from build123d import *

# Parameters (mm, degrees)
SALIENTE_EXTRUIR1_DEPTH = 5
CROQUIS3_W              = 50
CROQUIS3_H              = 80
CORTAR_EXTRUIR2_DEPTH   = 10
CHAFL_N1_SIZE           = 5
REDONDEO1_R             = 3
CROQUIS4_R              = 2.25
CORTAR_EXTRUIR3_DEPTH   = 5
CROQUIS5_R              = 30
CORTAR_EXTRUIR4_DEPTH   = 327.750669471


with BuildPart() as part:
    # Croquis1 → Saliente-Extruir1 (new body)
    with BuildSketch(Plane.XY):
        Polygon((0, 215), (0, 0), (246, 0), (246, 145), (216, 145), (216, 185), (176, 185), (176, 215), align=None)
        Polygon((-246, 145), (-246, 0), (0, 0), (0, 215), (-176, 215), (-176, 185), (-216, 185), (-216, 145), align=None)
        Polygon((0, 0), (-246, 0), (-246, -145), (-216, -145), (-216, -185), (-176, -185), (-176, -215), (176, -215), (176, -185), (216, -185), (216, -145), (246, -145), (246, 0), align=None)
    extrude(amount=SALIENTE_EXTRUIR1_DEPTH)

    # Croquis3 → Cortar-Extruir2 (cut)
    with BuildSketch(Plane.XY.offset(5)):
        with Locations((-221, 105)):
            Rectangle(CROQUIS3_W, CROQUIS3_H)
        with Locations((221, 105)):
            Rectangle(CROQUIS3_W, CROQUIS3_H)
    extrude(amount=-CORTAR_EXTRUIR2_DEPTH, mode=Mode.SUBTRACT)

    # Chaflán1
    chafl_n1_edges = [part.edges().sort_by_distance(p)[0] for p in [
        (-196, 65, 2.5),
        (-196, 145, 2.5),
        (196, 65, 2.5),
        (196, 145, 2.5),
    ]]
    chamfer(chafl_n1_edges, length=CHAFL_N1_SIZE)

    # Redondeo1
    redondeo1_edges = [part.edges().sort_by_distance(p)[0] for p in [
        (-196, 140, 2.5),
        (-196, 70, 2.5),
        (-201, 65, 2.5),
        (-201, 145, 2.5),
        (201, 65, 2.5),
        (196, 140, 2.5),
        (196, 70, 2.5),
        (201, 145, 2.5),
    ]]
    fillet(redondeo1_edges, radius=REDONDEO1_R)

    # Croquis4 → Cortar-Extruir3 (cut, symmetric)
    with BuildSketch(Plane.XY.offset(5)):
        with Locations((-146, 135)):
            Circle(CROQUIS4_R)
        with Locations((-96, 135)):
            Circle(CROQUIS4_R)
        with Locations((-146, 85)):
            Circle(CROQUIS4_R)
        with Locations((-96, 85)):
            Circle(CROQUIS4_R)
        with Locations((-46, 135)):
            Circle(CROQUIS4_R)
        with Locations((-46, 85)):
            Circle(CROQUIS4_R)
        with Locations((4, 135)):
            Circle(CROQUIS4_R)
        with Locations((4, 85)):
            Circle(CROQUIS4_R)
    extrude(amount=CORTAR_EXTRUIR3_DEPTH, both=True, mode=Mode.SUBTRACT)

    # Croquis5 → Cortar-Extruir4 (cut, through all)
    with BuildSketch(Plane.XY.offset(5)):
        with Locations((-121, 110)):
            Circle(CROQUIS5_R)
        with Locations((-21, 110)):
            Circle(CROQUIS5_R)
    extrude(amount=-CORTAR_EXTRUIR4_DEPTH, mode=Mode.SUBTRACT)


solid = part.part
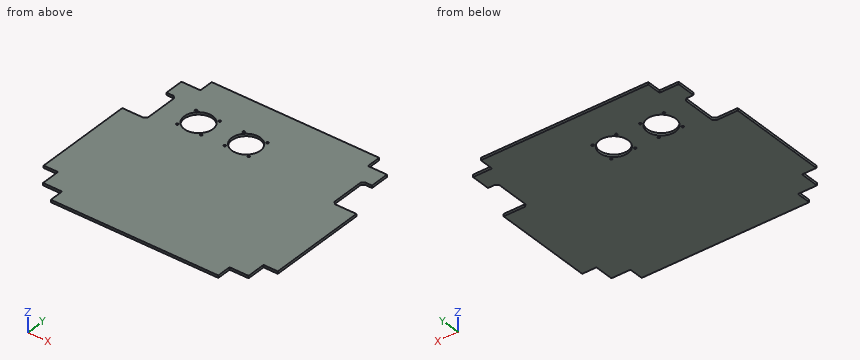
Can you work these out from the model? Positions are in its coordinate system, mm. Give positions to 0.01 mm unless a question says otherwise; leave off trailing zeros. Loops run counter-clockwise (first coordinate to the right, second up) from the corner with the lowest first, then second, coordinate; pieces in that order, holes last. Notation, with made-up numbers: (-11.75, 1) - (12.25, 1) arc R4 ccw to (12.25, 8) - close; hole circle Ø6 at (36, 66.5). An arc over 180 degrees is marked (long way). One line per item, written item: value.
(1) If we section it at B-B, the plane y = 110: List the corners of the cut face in (x, z) for me, plus the area to 3 significant figures.
Verdict:
outline: (-196, 0) - (-151, 0) - (-151, 5) - (-196, 5) - close; (-91, 0) - (-51, 0) - (-51, 5) - (-91, 5) - close; (9, 0) - (196, 0) - (196, 5) - (9, 5) - close
area: 1,360 mm^2
(2) If we section it at D-D, the plane x = -183.5: List the corners of the cut face in (y, z) for me.
Verdict:
outline: (-185, 0) - (185, 0) - (185, 5) - (-185, 5) - close
(3) I'm going to push flat-ended pins straight in: pin 1 (1.5 mm diameter, centred on x = 205, z = 2, fed in from -Y); pin 2 (1.5 mm diameter, centred on y = -161, z = 2.5, fed in from -X); pin 3 (10 mm diameter, centred on x = 182, y = 163.5, fed in from -Z); pin 4 (1.5 mm diameter, centred on x = 228.5, z = 3, fed in from -Y). Where does each tip first touch, or does it pass through?
Verdict:
pin 1: y = -185
pin 2: x = -216
pin 3: z = 0
pin 4: y = -145
(4) I need wall thicknesses on line 1 along Y through (x, z) = (4, 1.85); line 2 along X through (y, z) = (164, 4.4); line 3 along X through (y, z) = (101, 2.65). Which ranges of each line are inside material? Lowest first, please.
Verdict:
line 1: -215 to 82.75, 87.25 to 93.42, 126.58 to 132.75, 137.25 to 215
line 2: -216 to 216
line 3: -196 to -149.62, -92.38 to -49.62, 7.62 to 196
(5) If we section it at A-A, the plane x = -121: List the corners of the cut face in (y, z) for me.
Verdict:
outline: (-215, 0) - (80, 0) - (80, 5) - (-215, 5) - close; (140, 0) - (215, 0) - (215, 5) - (140, 5) - close
(6) If we section it at C-C, the plane z = 3.65: State how many separate pieces and enclosed holes the cut face has, plus the area to 3 significant figures.
Verdict:
separate pieces: 1
enclosed holes: 10
area: 185,000 mm^2
